from build123d import *

# Parameters (mm, degrees)
F0_W      = 26.593355462
F0_H      = 52.1527305245
F1_DEPTH  = 25.4
F2_DEPTH  = 25.4
F3_DEPTH  = 14.93277587
F6_D      = 25.4
F8_W      = 11.4883370697
F8_H      = 26.7024151981
F9_DEPTH  = 25.4
F10_W     = 13.3622530848
F10_H     = 31.2255714089
F11_DEPTH = 25.4
F12_R     = 7.1407496184
F13_DEPTH = 25.5624204874
F14_R     = 7.3663727873
F15_DEPTH = 24.5301295072


with BuildPart() as f1:
    # F0 (on Front) → F1 (new body)
    with BuildSketch(Plane.XZ):
        with Locations((6.2094768509, -19.6972563863)):
            Rectangle(F0_W, F0_H)
    extrude(amount=F1_DEPTH)

    # F2 (add): a face of the model
    f2_faces = [f1.faces().sort_by_distance(p)[0] for p in [
        (19.5061545819, -12.7, -19.6972563863),
    ]]
    extrude(f2_faces, amount=F2_DEPTH)

    # F3 (add): a face of the model
    f3_faces = [f1.faces().sort_by_distance(p)[0] for p in [
        (18.9094768509, -25.4, -19.6972563863),
    ]]
    extrude(f3_faces, amount=F3_DEPTH)

    # F6 (through all)
    with Locations(Plane.XZ.offset(40.33277587)):
        with Locations((17.0706212521, -18.9784392715)):
            Hole(F6_D / 2)

    # F8 (on face) → F9 (join)
    with BuildSketch(Plane.YZ.offset(44.9061545819)):
        with Locations((-19.0554484725, -22.4194079638)):
            Rectangle(F8_W, F8_H)
    extrude(amount=F9_DEPTH)

    # F10 (on face) → F11 (join)
    with BuildSketch(Plane(origin=(-7.0872008801, 0, 0), x_dir=(0, -1, 0), z_dir=(-1, 0, 0))):
        with Locations((21.9391398132, -22.3693735898)):
            Rectangle(F10_W, F10_H)
    extrude(amount=F11_DEPTH)

    # F12 (on face) → F13 (join)
    with BuildSketch(Plane.XZ.offset(24.7996170074)):
        with Locations((59.9011927843, -19.5363089442)):
            Circle(F12_R)
    extrude(amount=F13_DEPTH)

    # F14 (on face) → F15 (join)
    with BuildSketch(Plane.XZ.offset(28.6202663556)):
        with Locations((-22.8306427598, -22.3814845085)):
            Circle(F14_R)
    extrude(amount=F15_DEPTH)


solid = f1.part
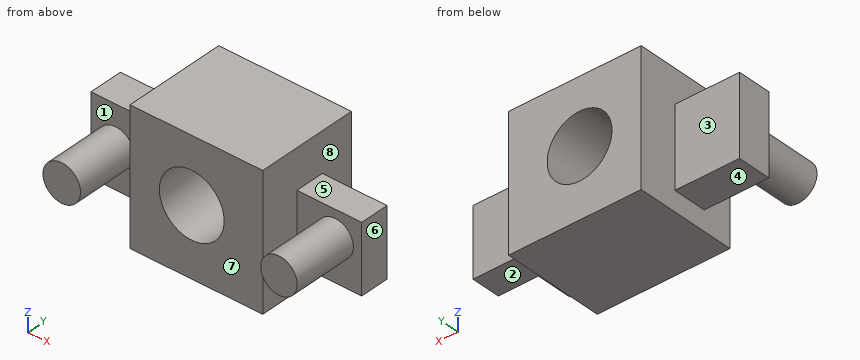
CAD build for the part. Positions are in the model's coordinates, mm. Face numbers are marked on the shaded views. A direction names the side the tool comes from. Round coordinates to 2 decimals unless told otherwise and drop trailing zeros. Write each loop counter-clockwise with the first axis right and the second up, starting at its lowest first coordinate (ties: lowest second). Pieces come first, ordered by that corner, then holes.
(1) Mould opens along X. For the marked faces 5, 6, 7 and 8 say: pulls with the +X half, pulls with the -X half, needs draft (parallel to the pull), parting line crosses it, or undercut.
(2) Slice it at B-B, the plane x = 10. Write the cut outline in (y, z), and give its area (3 significant figures).
(3) 3-axis set-ups, long thin cutter, end or side, ignore diameter. For the marked faces 1, 2, 3 and 4: which of +Z, -Z, +X, -X, +Y, -Y reach the whole face in a straight line?
(4) Slice it at D-D, the plane x = 62. Write the cut outline in (y, z), and give its area (3 significant figures).
(5) Slice it at A-A, the plane y = -35.5. Write the cut outline in (x, z), and give its area (3 significant figures).
(6) Drop flat-ended pins along their axis: P1, Ø12, axis at x = -17.5, y = -34, coming from the +Z side; P2, Ø7.5, axis at x = -18, z = -25.5, coming from the +Y side; P3, Ø20.5, axis at x = 17.07, z = -18.98, coming from the -Y side; P4, Ø20.5, axis at x = 60.5, z = -18.5, coming from the +Y side. Give the stop position or say it passes through.
(7) Slice it at C-C, the plane y = -21.5. Write the cut outline in (x, z), and give its area (3 significant figures).
(8) Probe line 1 along Z through (x, y) = (-23, -27); line 2 along Z through (x, y) = (19, -20); line 3 along X through (y, z) = (-19, -40.5). List the from-to ranges inside material, lowest first.
From the geometry:
1. face 5: needs draft
1. face 6: pulls with the +X half
1. face 7: undercut
1. face 8: undercut
2. outline: (-40.33, -45.77) - (0, -45.77) - (0, -29.53) - (-40.33, -29.53) - close; (-40.33, -8.43) - (0, -8.43) - (0, 6.38) - (-40.33, 6.38) - close
2. area: 1,250 mm2
3. face 1: -Y
3. face 2: -Z, +X, +Y, -Y
3. face 3: +Z, -Z, -X, +Y
3. face 4: -Z, -X, +Y, -Y
4. outline: (-50.36, -26.36) - (-24.8, -26.36) - (-24.8, -35.77) - (-13.31, -35.77) - (-13.31, -9.07) - (-24.8, -9.07) - (-24.8, -12.71) - (-50.36, -12.71) - close
4. area: 656 mm2
5. outline: circle Ø14.73 at (-22.83, -22.38); (-7.09, -45.77) - (44.91, -45.77) - (44.91, 6.38) - (-7.09, 6.38) - close; circle Ø14.28 at (59.9, -19.54); hole circle Ø25.4 at (17.07, -18.98)
5. area: 2,540 mm2
6. P1: stops at z = -6.76
6. P2: stops at y = -15.26
6. P3: passes through
6. P4: stops at y = -13.31
7. outline: (-32.49, -37.98) - (-7.09, -37.98) - (-7.09, -45.77) - (44.91, -45.77) - (44.91, -35.77) - (70.31, -35.77) - (70.31, -9.07) - (44.91, -9.07) - (44.91, 6.38) - (-7.09, 6.38) - (-7.09, -6.76) - (-32.49, -6.76) - close; hole circle Ø25.4 at (17.07, -18.98)
7. area: 3,680 mm2
8. line 1: z = -37.98 to -6.76
8. line 2: z = -45.77 to -31.53, -6.43 to 6.38
8. line 3: x = -7.09 to 44.91
